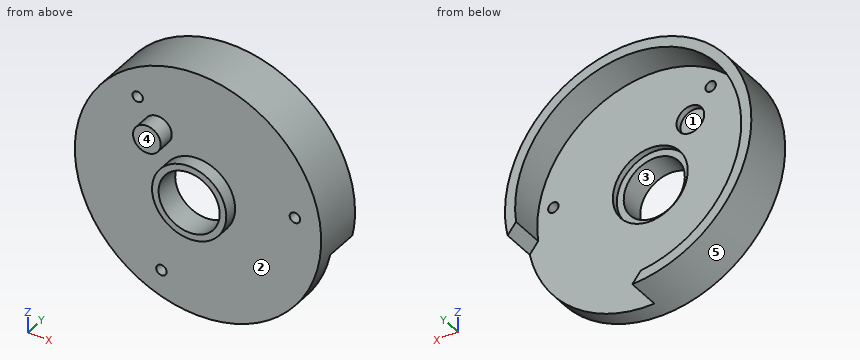
from build123d import *

# Parameters (mm, degrees)
SKETCH_1_R          = 36.5
SKETCH_1_R_2        = 11.1
SKETCH_1_R_3        = 4.1
EXTRUDE_1_DEPTH     = 5.3
SKETCH_2_R          = 36.5
SKETCH_2_R_2        = 33.5
EXTRUDE_1_2_DEPTH   = 10
SKETCH_4_R          = 4.1
EXTRUDE_3_DEPTH     = 5
SKETCH_5_R          = 4.1
EXTRUDE_4_DEPTH     = 3.5
CUT_EXTRUDE_1_DEPTH = 10
SKETCH_8_R          = 12
EXTRUDE_7_DEPTH     = 3.5
SKETCH_9_R          = 11
SKETCH_9_R_2        = 9.05
EXTRUDE_8_DEPTH     = 4
CUT_EXTRUDE_START   = -10
SKETCH_10_R         = 9.05
CUT_EXTRUDE_2_DEPTH = 10
SKETCH_11_R         = 1.55
CUT_EXTRUDE_3_DEPTH = 53.636394253


# Read off the part's stored shape, not the designer's step: the extrude step
with BuildPart() as part:
    # Sketch 1 → Extrude 1 (new body)
    with BuildSketch(Plane(origin=(0, 0, 0), x_dir=(1, 0, 0), z_dir=(0, 1, 0))):
        with Locations(Location((0, 0, 0), (0, 0, 270))):
            Circle(SKETCH_1_R)
        with Locations(Location((0, 0, 0), (0, 0, 270))):
            Circle(SKETCH_1_R_2, mode=Mode.SUBTRACT)
        with Locations(Location((-11.872537517, -15.152734173, 0), (0, 0, 270))):
            Circle(SKETCH_1_R_3, mode=Mode.SUBTRACT)
    extrude(amount=EXTRUDE_1_DEPTH)

    # Sketch 2 → Extrude 1 2 (add)
    with BuildSketch(Plane(origin=(0, 5.3, 0), x_dir=(1, 0, 0), z_dir=(0, 1, 0))):
        Circle(SKETCH_2_R)
        Circle(SKETCH_2_R_2, mode=Mode.SUBTRACT)
    extrude(amount=EXTRUDE_1_2_DEPTH)



with BuildPart() as body_2:
    # Sketch 4 → Extrude 3 (new body)
    with BuildSketch(Plane.XZ):
        with Locations(Location((-11.872537517, 15.152734173, 0), (0, 0, 90))):
            Circle(SKETCH_4_R)
    extrude(amount=EXTRUDE_3_DEPTH)


with BuildPart() as part_1:
    add(part.part)

    add(body_2.part)  # Extrude 4 merges body 2
    # Sketch 5 → Extrude 4 (add)
    with BuildSketch(Plane(origin=(0, 0, 0), x_dir=(1, 0, 0), z_dir=(0, 1, 0))):
        with Locations(Location((-11.872537517, -15.152734173, 0), (0, 0, 270))):
            Circle(SKETCH_5_R)
    extrude(amount=EXTRUDE_4_DEPTH)

    # Cut-Extrude 1 outline → Cut-Extrude 1 (cut)
    with BuildSketch(Plane(origin=(0, 5.3, 0), x_dir=(1, 0, 0), z_dir=(0, 1, 0))):
        with BuildLine():
            Line((33.216045924, 4.352504242), (35.712891568, 7.539189335))
            ThreePointArc((35.712891568, 7.539189335), (22.511564642, 28.731158302), (-1.223173568, 36.479498988))
            Line((-1.223173568, 36.479498988), (-3.720019212, 33.292813895))
            ThreePointArc((-3.720019212, 33.292813895), (20.661299055, 26.369693236), (33.216045924, 4.352504242))
        make_face()
    extrude(amount=CUT_EXTRUDE_1_DEPTH, mode=Mode.SUBTRACT)

    # Sketch 8 → Extrude 7 (add)
    with BuildSketch(Plane.XZ):
        Circle(SKETCH_8_R)
    extrude(amount=-EXTRUDE_7_DEPTH)

    # Sketch 9 → Extrude 8 (add)
    with BuildSketch(Plane.XZ):
        with Locations(Location((0, 0, 0), (0, 0, 90))):
            Circle(SKETCH_9_R)
        with Locations(Location((0, 0, 0), (0, 0, 270))):
            Circle(SKETCH_9_R_2, mode=Mode.SUBTRACT)
    extrude(amount=EXTRUDE_8_DEPTH)

    # Sketch 10 → Cut-Extrude 2 (cut)
    with BuildSketch(Plane.XZ.offset(4).offset(CUT_EXTRUDE_START)):
        with Locations(Location((0, 0, 0), (0, 0, 270))):
            Circle(SKETCH_10_R)
    extrude(amount=CUT_EXTRUDE_2_DEPTH, mode=Mode.SUBTRACT)

    # Sketch 11 → Cut-Extrude 3 (cut, through all)
    with BuildSketch(Plane(origin=(0, 5.3, 0), x_dir=(1, 0, 0), z_dir=(0, 1, 0))):
        with Locations(Location((-17.885900675, -22.827495637, 0), (0, 0, 270))):
            Circle(SKETCH_11_R)
        with Locations(Location((-10.826240789, 26.903392172, 0), (0, 0, 270))):
            Circle(SKETCH_11_R)
        with Locations(Location((28.712141464, -4.075896535, 0), (0, 0, 270))):
            Circle(SKETCH_11_R)
    extrude(amount=-CUT_EXTRUDE_3_DEPTH, mode=Mode.SUBTRACT)


solid = part_1.part
Source: CAD feature listing. Evaluate the final solid. Frame: model axes, mm. Face numbers are marked on the shaded views. A direction names the side the tool comes from. Coordinates: 2 decimals unless noted, no trailing zeros. Order: outer loops, then holes, each group sorted by start corner. A loop starts at its lowest first (then second) coordinate and runs counter-clockwise, first axis right, second up. Notation, with made-up numbers: M 33,35 L 52,35 A23 cw 52,62 Z; hole C 36.25,-19.75 d8. An arc over 180 degrees is marked long. Write each question's results on one line, items separated by ' | '. Start each with the question number.
Item 1: Cut plane A-A (x = -2.5). Return loops of the section in (y, z).
Item 2: Cut plane B-B (y = -2.75). Return loops of the section in (x, z).
Item 3: Set-up query: the marked faces 1 and 2. Return all of +Z, -Z, +X, -X, +Y, -Y with unobstructed straight access to the full face (end or side cutting, diameter ignored); none if empty.
Item 4: Line query: probe 1 along X at (y, z) = (8, 0); probe 2 along Z at (x, y) = (0, 13); probe 3 along Z at (x, y) = (-21, 13.25). Output: solid intervals per line, ascending.
Item 5: Cut plane D-D (y = 7). Return loops of the section in (x, z), and give its area (3 significant figures).
Item 6: Draft query along Z for the marked faces 3, 4 and 5. Return one class per face: pulls with the +Z half, pulls with the -Z half, needs draft (parallel to the pull), parting line crosses it, or undercut.
Item 7: First-contact query: pin 1 Ø3 at (x, y) = (2, 2.5) entering from -Z; pin 2 Ø12 at (x, y) = (27.5, 8.5) entering from +Z; pin 3 Ø2.5 at (x, z) = (-17.89, 22.83) entering from -Y; pin 4 Ø2 at (y, z) = (8.5, 6) entering from -X. Flat tips, straight axial feed; report the tip coordinate or a pass-through.
Item 8: Cut plane C-C (x = -27). Return loops of the section in (y, z).
Checked values:
1) outline: M -4,-10.71 L 0,-10.71 L 0,-36.41 L 15.3,-36.41 L 15.3,-34.85 L 5.3,-34.85 L 5.3,-10.81 L 3.5,-10.81 L 3.5,-8.7 L -4,-8.7 Z; M -4,8.7 L 3.5,8.7 L 3.5,10.81 L 5.3,10.81 L 5.3,33.41 L 15.3,33.41 L 15.3,36.41 L 0,36.41 L 0,10.71 L -4,10.71 Z
2) outline: C -11.87,15.15 d8.2; C 0,0 d22; hole C 0,0 d18.1
3) face 1: +Y | face 2: -Y
4) probe 1: x = -36.5 to -33.5, 33.5 to 36.5 | probe 2: z = 33.5 to 36.5 | probe 3: z = -29.85 to -26.1, 26.1 to 29.85
5) outline: M -3.72,-33.29 A33.5 cw long 33.22,-4.35 L 35.71,-7.54 A36.5 ccw long -1.22,-36.48 Z | area: 505 mm2
6) face 3: undercut | face 4: needs draft | face 5: parting line crosses it
7) pin 1: stops at z = -36.5 | pin 2: stops at z = 29.5 | pin 3: passes through | pin 4: stops at x = -36.16
8) outline: M 0,-24.56 L 15.3,-24.56 L 15.3,-19.83 L 5.3,-19.83 L 5.3,19.83 L 15.3,19.83 L 15.3,24.56 L 0,24.56 Z
